Check sheet for the modelled part. Datum: model origin and axes. Units: mm. Face numbers are marked on the shaded views. A direction names the side the tool comes from. Round coordinates to 2 decimals unless told otherwise and drop trailing zeros. Loops run counter-clockwise (first coordinate to the right, second up) from the corner with the lowest first, then second, coordinate; pieces in that order, holes last. Notation, with made-up numbers: (58.25, -23) - (62.25, -23) arc R26 cw to (62.25, 14) - close; hole circle Ø8 at (-35.75, 24.25). An arc over 180 degrees is marked (long way). Put each result on its own line as item: value. Start each with the question number.
Item 1: Section check C-C, the plane y = 17.5. Record the cut outline in (x, z), and give its area (3 significant figures).
Item 2: Gauge pin test, flat ends, axial feed: pin 1 Ø1 at (x, y) = (28, 15) entering from -Z; pin 2 Ø3 at (x, y) = (-29, 56.5) entering from -Z; pin 3 Ø1.5 at (y, z) = (41.5, 4) entering from -X; pin 4 Ø4 at (x, z) = (-31, -30.5) entering from +Y. Record the tip position at first contact, or that the pin passes through.
Item 3: Section check D-D, the plane y = 5.5. Record the cut outline in (x, z).
Item 4: Draft check along Z on the marked faces 1, 2 and 3. Enter one of: pulls with the +Z half, pulls with the -Z half, needs draft (parallel to the pull), parting line crosses it, or undercut.
Item 5: Material ranges on line 1 along X through (y, z) = (24.5, 0); line 2 along Y through (x, z) = (-20.5, -26); line 3 along X through (y, z) = (6, -33), recorded low to high.
Item 6: Tool access check on the marked faces 4, 5 and 6. Record the directions out of +Z, -Z, +X, -X, +Y, -Y that give a thin tool (end or side, any length) a straight path to the whole face; none if there is none.
Item 7: Section check A-A, the plane y = 46. Record the cut outline in (x, z), and give its area (3 significant figures).
Item 8: Section check B-B, the plane x = 0. Give the number of separate pieces and of enclosed holes in the cut face, and give its area (3 significant figures).
from build123d import *

# Parameters (mm, degrees)
PATTERN_CIRCULAR_1_COUNT = 8


with BuildPart() as part:
    # Эскиз1 → Повернуть1 (revolve)
    with BuildSketch(Plane.XY, mode=Mode.PRIVATE) as revolve_1_sk:
        Polygon((-42, 0), (-60, 0), (-60, 9), (-61.5, 9), (-62.5, 10), (-62.5, 28), (-61.5, 29), (-57, 29), (-57, 37), (-60, 40), (-60, 67), (-57, 70), (-46.5, 70), (-46.5, 35), (-31.5, 35), (-31.5, 10), (-42, 10), align=None)
    revolve(revolve_1_sk.sketch.rotate(Axis((0, 0, 0), (0, 1, 0)), 270), axis=Axis((0, 0, 0), (0, 1, 0)))

    # Эскиз5 → Вырез-Повернуть1 (revolve, cut)
    with BuildSketch(Plane.XY):
        Polygon((-43, 0), (-46, 0), (-46, 30), (-50, 30), (-50, 70), (-43, 70), align=None)
    cut_revolve_1 = revolve(axis=Axis((-43, 84.512066433, 0), (0, -1, 0)), mode=Mode.SUBTRACT)

    # Круговой массив1: Вырез-Повернуть1 ×8 about axis, 2 skipped
    pattern_circular_1_axis = Axis((0, 0, 0), (0, -1, 0))
    add([cut_revolve_1.rotate(pattern_circular_1_axis, i * 360 / PATTERN_CIRCULAR_1_COUNT) for i in range(1, PATTERN_CIRCULAR_1_COUNT) if i not in (6, 7)], mode=Mode.SUBTRACT)


solid = part.part
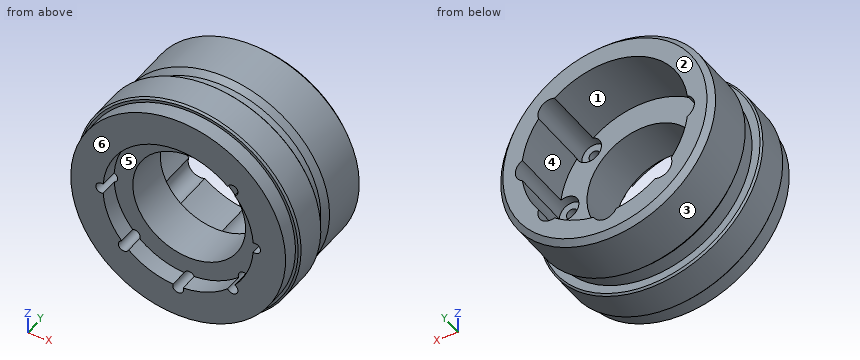
Check result:
1. outline: circle Ø125 at (0, 0); hole circle Ø6 at (-43, 0); hole circle Ø6 at (-30.41, -30.41); hole circle Ø63 at (0, 0); hole circle Ø6 at (0, -43); hole circle Ø6 at (30.41, -30.41); hole circle Ø6 at (30.41, 30.41); hole circle Ø6 at (43, 0)
1. area: 8,980 mm²
2. pin 1: z = -56.12
2. pin 2: z = -53.33
2. pin 3: x = -59.91
2. pin 4: through
3. outline: circle Ø120 at (0, 0); hole (-41.91, -2.79) arc R42 ccw to (-31.61, -27.66) arc R3 ccw (long way) to (-27.66, -31.61) arc R42 ccw to (-2.79, -41.91) arc R3 ccw (long way) to (2.79, -41.91) arc R42 ccw to (27.66, -31.61) arc R3 ccw (long way) to (31.61, -27.66) arc R42 ccw to (41.91, -2.79) arc R3 ccw (long way) to (41.91, 2.79) arc R42 ccw to (31.61, 27.66) arc R3 ccw (long way) to (27.66, 31.61) arc R42 ccw to (-41.91, 2.79) arc R3 ccw (long way) to start
4. face 1: undercut
4. face 2: needs draft
4. face 3: parting line crosses it
5. line 1: -62.5 to -46, -40 to -31.5, 31.5 to 40, 46 to 62.5
5. line 2: 10 to 35
5. line 3: -50.11 to -31.91, -28.9 to -25.98, 25.98 to 28.9, 31.91 to 50.11
6. face 4: +Y
6. face 5: -Y
6. face 6: +Z, -Z, +X, -X, -Y
7. outline: circle Ø120 at (0, 0); hole (-46.07, -6.29) arc R46.5 ccw to (-37.03, -28.13) arc R7 ccw to (-28.13, -37.03) arc R46.5 ccw to (-6.29, -46.07) arc R7 ccw to (6.29, -46.07) arc R46.5 ccw to (28.13, -37.03) arc R7 ccw to (37.03, -28.13) arc R46.5 ccw to (46.07, -6.29) arc R7 ccw to (46.07, 6.29) arc R46.5 ccw to (37.03, 28.13) arc R7 ccw to (28.13, 37.03) arc R46.5 ccw to (-46.07, 6.29) arc R7 ccw to start
7. area: 4,330 mm²
8. separate pieces: 3
8. enclosed holes: 0
8. area: 2,410 mm²
